Source: CAD feature listing. Evaluate the final solid. Frame: model axes, mm. A direction names the side the tool comes from. Round coordinates to 2 decimals unless told otherwise and drop trailing zeros. Order: outer loops, then holes, each group sorted by start corner. A loop starts at its lowest first (then second) coordinate and runs counter-clockwise, first axis right, second up. Notation, with made-up numbers: (22.25, 82) -> (29.25, 82) arc R6 cw to (29.25, 87) -> close; hole circle Ø10 at (74, 25.5). An arc over 180 degrees is marked (long way). Answer as CSV lines item,"result".
from build123d import *

# Parameters (mm, degrees)
BOSS_EXTRUDE1_DEPTH = 20
SKETCH2_W           = 20
SKETCH2_H           = 3.175
CUT_EXTRUDE2_DEPTH  = 490.591666596


with BuildPart() as part:
    # Sketch1 → Boss-Extrude1 (new body)
    with BuildSketch(Plane(origin=(0, 0, 0), x_dir=(1, 0, 0), z_dir=(0, 1, 0))):
        Polygon((320, 245), (270, 175), (320, 215), (320, 105), (370, 35), (320, 75), (320, 0), (0, 0), (0, 320), (320, 320), align=None)
    extrude(amount=BOSS_EXTRUDE1_DEPTH)

    # Sketch2 → Cut-Extrude2 (cut, through all)
    with BuildSketch(Plane(origin=(0, 20, 0), x_dir=(1, 0, 0), z_dir=(0, 1, 0))):
        with Locations((225, 233.4125)):
            Rectangle(SKETCH2_W, SKETCH2_H)
        with Locations((95, 233.4125)):
            Rectangle(SKETCH2_W, SKETCH2_H)
        with Locations((95, 86.5875)):
            Rectangle(SKETCH2_W, SKETCH2_H)
        with Locations((225, 86.5875)):
            Rectangle(SKETCH2_W, SKETCH2_H)
    extrude(amount=-CUT_EXTRUDE2_DEPTH, mode=Mode.SUBTRACT)


solid = part.part
1. Section query D-D on z = -161. Return loops of the section in (x, y), and give its area (3 significant figures).
Results below:
outline,"(0, 0) -> (320, 0) -> (320, 20) -> (0, 20) -> close"
area,"6,400 mm2"
2. Mould query, pull axis Z, two halves, no side actions, for faces 1 (the flat face through (295, 10, -210)), 2 (the flat face through (345, 10, -70)), 3 (the flat face through (0, 10, -158)). Classes: released by +Z, released by -Z, zero draft, split by the parting line, or undercut.
Results below:
face 1,"undercut"
face 2,"released by -Z"
face 3,"zero draft"
3. Pin query (flat end, axial travel): pin 1 (8 mm diameter, centred on y = 8, z = -62, fed in from +X); pin 2 (10 mm diameter, centred on y = 15, z = -155.5, fed in from +X); pin 3 (1.6 mm diameter, centred on y = 5.5, z = -86, fed in from +X). Return the tip coordinate at first contact, or that it passes through.
Results below:
pin 1,"x = 353.57"
pin 2,"x = 320"
pin 3,"x = 334.14"
4. Section query A-A on z = -49. Return loops of the section in (x, y), and give its area (3 significant figures).
Results below:
outline,"(0, 0) -> (320, 0) -> (320, 20) -> (0, 20) -> close; (352.5, 0) -> (360, 0) -> (360, 20) -> (352.5, 20) -> close"
area,"6,550 mm2"
5. Section query B-B on y = 7.25. Return loops of the section in (x, z) (3 decimals).
Results below:
outline,"(0, -320) -> (320, -320) -> (320, -245) -> (270, -175) -> (320, -215) -> (320, -105) -> (370, -35) -> (320, -75) -> (320, 0) -> (0, 0) -> close; hole (85, -235) -> (105, -235) -> (105, -231.825) -> (85, -231.825) -> close; hole (85, -88.175) -> (105, -88.175) -> (105, -85) -> (85, -85) -> close; hole (215, -235) -> (235, -235) -> (235, -231.825) -> (215, -231.825) -> close; hole (215, -88.175) -> (235, -88.175) -> (235, -85) -> (215, -85) -> close"
6. Line query: L1, parallel to Z at x = 103, y = 18.5 (3 decimals); L2, parallel to X at y = 8.25, z = -127; L3, parallel to X at y = 14.5, z = -39.5 (3 decimals). Output: solid intervals per line, ascending. Write a range as [from, to].
Results below:
L1,"[-320, -235], [-231.825, -88.175], [-85, 0]"
L2,"[0, 320]"
L3,"[0, 320], [364.375, 366.786]"
7. Reachability of faces 4 (the flat face through (225, 10, -88.175)), 5 (the flat face through (320, 10, -38)), 6 (the flat face through (320, 10, -161)) from +Z, -Z, +X, -X, +Y, -Y: full face, straight path, thin tool, end or side. Return the list, or none.
Results below:
face 4,"+Y, -Y"
face 5,"+Z, +Y, -Y"
face 6,"-Z, +X, +Y, -Y"
8. Section query C-C on x = 329. Return loops of the section in (y, z).
Results below:
outline,"(0, -92.4) -> (20, -92.4) -> (20, -67.8) -> (0, -67.8) -> close"
